Geometry check sheet. Reference: the model listing, model coordinates, mm. A direction names the side the tool comes from. Coordinates: 2 decimals unless noted, no trailing zeros. Write each loop counter-clockwise with the first axis right and the second up, starting at its lowest first coordinate (ties: lowest second). Pieces come first, ordered by that corner, then holes. Notation, with made-up numbers: (52.5, -3) -> (74.5, -3) arc R17 ccw to (74.5, 17) -> close; hole circle Ø1 at (32, -38). An arc over 180 degrees is marked (long way). Answer in a Markdown table with one row per item. Add a question column.
1. Cross-section at B-B on z = 21. Record the cut outline in (x, y), and give its area (3 significant figures).
2. Cross-section at A-A on y = -3.75. Record the cut outline in (x, z), and give its area (3 significant figures).
3. Mould release check, pull along Z, two halves, no side actions. Record for faces 3 (the cylindrical face through (-30.7, -3.1, -18.3)), 4 (the cylindrical face through (-27, -3, -26)), 5 (the flat face through (-11, -3, 27.691)): pulls with the +Z half, pulls with the -Z half, needs draft (parallel to the pull), parting line crosses it, or undercut.
4. Depth check by flat-ended pin: P1, Ø1, axis at y = -3, z = 8, coming from the -X side; P2, Ø1, axis at y = -2, z = -1, coming from the -X side; P3, Ø1, axis at y = -3.5, z = 7.5, coming from the +X side. Enter the tip coordinate at first touch or a pass-through.
5. Scan lines: L1, parallel to X at y = -4.25, z = 25; L2, parallel to Z at x = -35, y = -5.5; L3, parallel to X at y = -5.75, z = -7.5. Record each from-to range of solid material in increasing order. Write a range as from..to.
6. Set-up check for faces 1 (the flat face through (-18.256, -3, 22)), 2 (the flat face through (-18, -6.35, 0)): record each of +Z, -Z, +X, -X, +Y, -Y from which the full face is reachable in a straight line by a thin tool's end or side.
7. Cross-section at C-C on x = -11.5. Record the cut outline in (y, z), and give its area (3 significant figures).
```python
from build123d import *

# Parameters (mm, degrees)
F1_DEPTH = 6.35


with BuildPart() as f1:
    # F0 (on Front) → F1 (new body)
    with BuildSketch(Plane.XZ):
        with BuildLine():
            Line((-4.778545, 27.691057), (-18.256493, 27.691057))
            Line((-18.256493, 27.691057), (-18.256493, 15.928484))
            ThreePointArc((-18.256493, 15.928484), (-25.850649, 5.196476), (-29.774012, -7.351608))
            ThreePointArc((-29.774012, -7.351608), (-30.768982, -18.490309), (-37.125621, -27.691057))
            ThreePointArc((-37.125621, -27.691057), (-26.863912, -25.947249), (-18.256493, -20.094397))
            ThreePointArc((-18.256493, -20.094397), (-8.258358, -3.30237), (-4.778545, 15.928484))
            Line((-4.778545, 15.928484), (-4.778545, 27.691057))
        make_face()
    extrude(amount=F1_DEPTH)


solid = f1.part
```
Results found:
| question | item | result |
|---|---|---|
| 1 | outline | (-18.26, -6.35) -> (-4.78, -6.35) -> (-4.78, 0) -> (-18.26, 0) -> close |
| 1 | area | 85.6 mm^2 |
| 2 | outline | (-37.13, -27.69) arc R24.46 ccw to (-18.26, -20.09) arc R54.88 ccw to (-4.78, 15.93) -> (-4.78, 27.69) -> (-18.26, 27.69) -> (-18.26, 15.93) arc R42.2 ccw to (-29.77, -7.35) arc R21.94 cw to start |
| 2 | area | 887 mm^2 |
| 3 | face 3 | undercut |
| 3 | face 4 | pulls with the -Z half |
| 3 | face 5 | pulls with the +Z half |
| 4 | P1 | stops at x = -24.62 |
| 4 | P2 | stops at x = -28.48 |
| 4 | P3 | stops at x = -5.35 |
| 5 | L1 | x = -18.26..-4.78 |
| 5 | L2 | z = -27.7..-25.6 |
| 5 | L3 | x = -29.75..-10.03 |
| 6 | face 1 | +Z, -X, +Y, -Y |
| 6 | face 2 | +Z, -Z, +X, -X, -Y |
| 7 | outline | (-6.35, -10.39) -> (0, -10.39) -> (0, 27.69) -> (-6.35, 27.69) -> close |
| 7 | area | 242 mm^2 |
